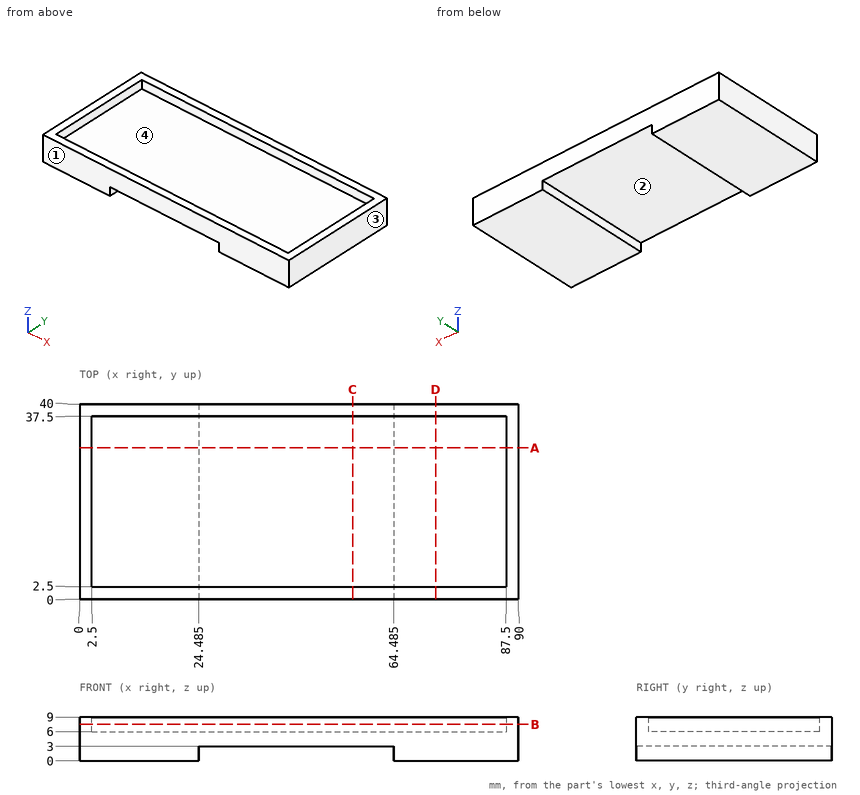
Drawing for the job (mm, zero at the part's lowest x, y, z). Give positions to 0.01 mm unless a question says otherwise; leave off trailing zeros. Write each loop counter-clockwise with the first axis right and the second up, starting at its lowest first coordinate (ties: lowest second). Pieces come first, ordered by that corner, then holes. Notation, with made-up numbers: (-32.75, 83) -> (23.25, 83) arc R24 cw to (23.25, 119) -> close; hole circle Ø8 at (25.25, -16.75). An arc over 180 degrees is marked (long way). Put each result on its own line as item: value. Start each with the question number.
Item 1: Cut at D-D (x = 73). List the corners of the cut face in (y, z), then the cut area to 3 significant figures.
Item 2: Cut at B-B (z = 7.5). List the corners of the cut face in (x, y), then the cut area to 3 significant figures.
Item 3: Pin check, flat tips, straight feed: pin 1 Ø2 at (x, y) = (29, 26.5) entering from -Z; pin 2 Ø17.5 at (x, y) = (50.5, 17.5) entering from +Z. Stop position of each tip, or through.
Item 4: Wall check: L1, parallel to Y at x = 13, z = 6.5; L2, parallel to X at y = 29, z = 8.75; L3, parallel to X at y = 28.5, z = 2.25 (1 decimal). Give the ranges that are in metal, low to high. Write a range as [from, to].
Item 5: Cut at A-A (y = 31). List the corners of the cut face in (x, z) (1 decimal), then the cut area to 3 significant figures.
Item 6: Pull direction X, two halves, no side cores. Call the marked faces 1, 2, 3 and 4: pulls with the +X half, pulls with the -X half, needs draft (parallel to the pull), parting line crosses it, or undercut.
Item 7: Cut at C-C (x = 56). List the corners of the cut face in (y, z), then the cut area to 3 significant figures.
Answer list:
1. outline: (0, 0) -> (40, 0) -> (40, 9) -> (37.5, 9) -> (37.5, 6) -> (2.5, 6) -> (2.5, 9) -> (0, 9) -> close
1. area: 255 mm2
2. outline: (0, 0) -> (90, 0) -> (90, 40) -> (0, 40) -> close; hole (2.5, 2.5) -> (87.5, 2.5) -> (87.5, 37.5) -> (2.5, 37.5) -> close
2. area: 625 mm2
3. pin 1: stops at z = 3
3. pin 2: stops at z = 6
4. L1: y = [0, 2.5], [37.5, 40]
4. L2: x = [0, 2.5], [87.5, 90]
4. L3: x = [0, 24.5], [64.5, 90]
5. outline: (0, 0) -> (24.5, 0) -> (24.5, 3) -> (64.5, 3) -> (64.5, 0) -> (90, 0) -> (90, 9) -> (87.5, 9) -> (87.5, 6) -> (2.5, 6) -> (2.5, 9) -> (0, 9) -> close
5. area: 435 mm2
6. face 1: needs draft
6. face 2: undercut
6. face 3: pulls with the +X half
6. face 4: undercut
7. outline: (0, 3) -> (40, 3) -> (40, 9) -> (37.5, 9) -> (37.5, 6) -> (2.5, 6) -> (2.5, 9) -> (0, 9) -> close
7. area: 135 mm2
